```python
from build123d import *

# Parameters (mm, degrees)
F0_W           = 304.8
F0_H           = 203.2
F1_DEPTH       = 25.4
F2_W           = 76.2
F2_H           = 12.7
F3_DEPTH       = 378.206
F6_D           = 5.25
F6_CSINK_D     = 11.2
F6_CSINK_ANGLE = 90
F7_W           = 228.6
F7_H           = 50.8
F8_DEPTH       = 50.8
F9_T           = -2.54
F4_R           = 25.4
F13_DEPTH      = 25.4


# Not quite as in the source:
# - a shell that OpenCascade refuses in one call is made with other operations: the cavity is built on its own and cut out
# - the program builds the solid bodies; features that only make, move or delete a surface that nothing else refers to are left out


with BuildPart() as f1:
    # F0 (on Top) → F1 (new body)
    with BuildSketch(Plane.XY):
        Rectangle(F0_W, F0_H)
    extrude(amount=F1_DEPTH)

    # F2 (on face) → F3 (cut)
    with BuildSketch(Plane(origin=(-152.4, 0, 0), x_dir=(0, -1, 0), z_dir=(-1, 0, 0))):
        with Locations((-57.15, 12.7)):
            Rectangle(F2_W, F2_H)
    extrude(amount=-F3_DEPTH, mode=Mode.SUBTRACT)

    # F6 (through all)
    with Locations(Plane(origin=(-152.4, 0, 0), x_dir=(0, -1, 0), z_dir=(-1, 0, 0))):
        with Locations((0, 12.7)):
            CounterSinkHole(F6_D / 2, F6_CSINK_D / 2, counter_sink_angle=F6_CSINK_ANGLE)

    # F7 (on face) → F8 (join)
    with BuildSketch(Plane.XY.offset(25.4)):
        Rectangle(F7_W, F7_H)
    extrude(amount=F8_DEPTH)

    # F9: a shell. OpenCascade refuses it in one call, so the cavity is built on its own and cut out:
    # the body offset inwards by the wall thickness, plus a prism from it out through each open face.
    f9_core = offset(f1.part, amount=F9_T, kind=Kind.INTERSECTION, mode=Mode.PRIVATE)
    f9_exits = [f9_core.faces().sort_by_distance(p)[0] for p in [
        (0, -22.86, 48.26),
    ]]
    add(f9_core, mode=Mode.SUBTRACT)
    extrude(f9_exits, amount=-F9_T, mode=Mode.SUBTRACT)

    # F4 (on face) → F13 (cut)
    with BuildSketch(Plane.XY.offset(25.4)):
        with Locations((-88.3831381798, 51.9134663045)):
            Circle(F4_R)
    extrude(amount=-F13_DEPTH, mode=Mode.SUBTRACT)


solid = f1.part
```
The model under review builds one solid part; all positions refer to its coordinate system, in mm. A direction names the side the tool comes from. Give positions to 0.01 mm unless a question says otherwise; leave off trailing zeros. Write each loop counter-clockwise with the first axis right and the second up, starting at its lowest first coordinate (ties: lowest second). Pieces come first, ordered by that corner, then holes. Notation, with made-up numbers: M 80,54 L 95,54 A21 cw 95,60 Z; hole C -36.5,38.25 d1. An arc over 180 degrees is marked long. Write item = value, one per line. Start each with the question number.
Q1. Clearance check with flat-ended pins moving along their axes: pin 1 (1.5 mm diameter, centred on x = 106, y = 34, fed in from +Z); pin 2 (6 mm diameter, centred on x = 42.5, z = 38.5, fed in from +Y); pin 3 (2 mm diameter, centred on x = 59.5, z = 37, fed in from -Y). State where each tip first meets the part, or that it passes through.
Q2. We need section A-A (x = 72). State the section outline as (y, z) points (3 decimals), plus the area to 3 significant figures.
Q3. For line 1 (Z direction, x = -40.5, y = 22); line 2 (Y direction, x = -40.5, z = 12.7) (3 decimals); line 3 (Z direction, x = 57, y = 47), list the stretches that pass through material, from the lowest coordinate up.
Q4. Mouldability with a two-part tool opening along Y and no side actions: class faces 4 (the face through (-2, 25.4, 50)), 5 (the face through (-107.104, 69.08, 20.338)), 6 (the face through (-1, -25.4, 75)), 7 (the face through (-2, 95.25, 13)) as released by +Y, released by -Y, zero draft, split by the parting line, or undercut.
Q5. We need section B-B (y = 64). Give the number of separate pieces and of enclosed holes in the cut face, plus the area to 3 significant figures.
Q6. Machinability: for faces 1 (the face through (-2, 58, 3.81)), 2 (the face through (-2, 101.6, 13)), 3 (the face through (-2, 58, 19.05)), which of the approach directions +Z, -Z, +X, -X, +Y, -Y give a long, thin tool a straight path to every point of the face, cutting with its end or side? Answer none if there is none.
Q7. We need section C-C (z = 56.5). State the section outline as (x, y) points.
Result set:
q1.pin_1 = 25.4
q1.pin_2 = 25.4
q1.pin_3 = 22.86
q2.outline = M -101.6,0 L 101.6,0 L 101.6,25.4 L 25.4,25.4 L 25.4,76.2 L -25.4,76.2 L -25.4,73.66 L 22.86,73.66 L 22.86,22.86 L 99.06,22.86 L 99.06,2.54 L -99.06,2.54 L -99.06,22.86 L -25.4,22.86 L -25.4,25.4 L -101.6,25.4 Z; C 0,12.7 d10.33; M 16.51,3.81 L 97.79,3.81 L 97.79,21.59 L 16.51,21.59 Z; hole C 0,12.7 d5.25; hole M 19.05,6.35 L 95.25,6.35 L 95.25,19.05 L 19.05,19.05 Z
q2.area = 1,800 mm2
q3.line_1 = 0 to 2.54, 3.81 to 6.35, 19.05 to 21.59, 73.66 to 76.2
q3.line_2 = -101.6 to -99.06, -5.165 to -2.625, 2.625 to 5.165, 16.51 to 19.05, 95.25 to 97.79, 99.06 to 101.6
q3.line_3 = 0 to 2.54, 3.81 to 6.35, 19.05 to 21.59, 22.86 to 25.4
q4.face_4 = released by +Y
q4.face_5 = undercut
q4.face_6 = released by -Y
q4.face_7 = undercut
q5.separate_pieces = 4
q5.enclosed_holes = 0
q5.area = 2,660 mm2
q6.face_1 = none
q6.face_2 = +Z, -Z, +X, -X, +Y
q6.face_3 = +X, -X
q7.outline = M -114.3,-25.4 L -111.76,-25.4 L -111.76,22.86 L 111.76,22.86 L 111.76,-25.4 L 114.3,-25.4 L 114.3,25.4 L -114.3,25.4 Z
